Answer from the drawing. Dimensions are ordinates in mm from the lowest x, y and z of the part. A direction names the side the tool comes from. Give positions to 0.01 mm unless a question says otherwise; leave off trailing zeros. Write each loop counter-clockwise with the first axis right and the second up, starting at its lowest first coordinate (ties: lowest second). Pieces come first, ordered by that corner, then holes. Notation, with made-up numbers: (-18, 64.5) -> (-10, 64.5) arc R25 cw to (-10, 89.5) -> close; hole circle Ø4 at (73.25, 89.5). An arc over 180 degrees is marked (long way). Put each result on its own line as item: value. Start each with the question number.
1) A cutting plane is placed at C-C (y = 32). Write down the section's boundary in (x, z), then the cut area to 3 significant figures.
2) For a pull along Z with two mould halves and no side action, classify the marked faces 1, 2 and 3 as released by +Z, released by -Z, zero draft, split by the parting line, or undercut.
3) A cutting plane is placed at B-B (x = 54). Write down the section's boundary in (y, z), then the cut area to 3 significant figures.
4) A cutting plane is placed at D-D (z = 6). Give the number of separate pieces and of enclosed holes in the cut face, then the cut area to 3 significant figures.
5) A cutting plane is placed at A-A (y = 24.5). Write down the section's boundary in (x, z), then the cut area to 3 significant figures.
6) Find the intervals of material crossed by line 1 along Z through (x, y) = (54, 3); line 2 along X through (y, z) = (20, 8); line 3 along Y through (x, z) = (39.55, 15), in increasing order. Write a range as from..to.
7) For the marked faces 4, 5, 6 and 7, determine the directions among +Z, -Z, +X, -X, +Y, -Y from which every point of the face is accessible in a straight line to the end or side of a thin tool.
8) Flat-ended cylindrical pins translate along their axes: pin 1 Ø13 at (y, z) = (36, 15) entering from +X; pin 2 Ø6 at (y, z) = (13.5, 11.5) entering from -X; pin 3 Ø6.5 at (x, z) = (50.5, 19) entering from +Y. Find the tip coordinate at first contact, or state that the pin passes through.
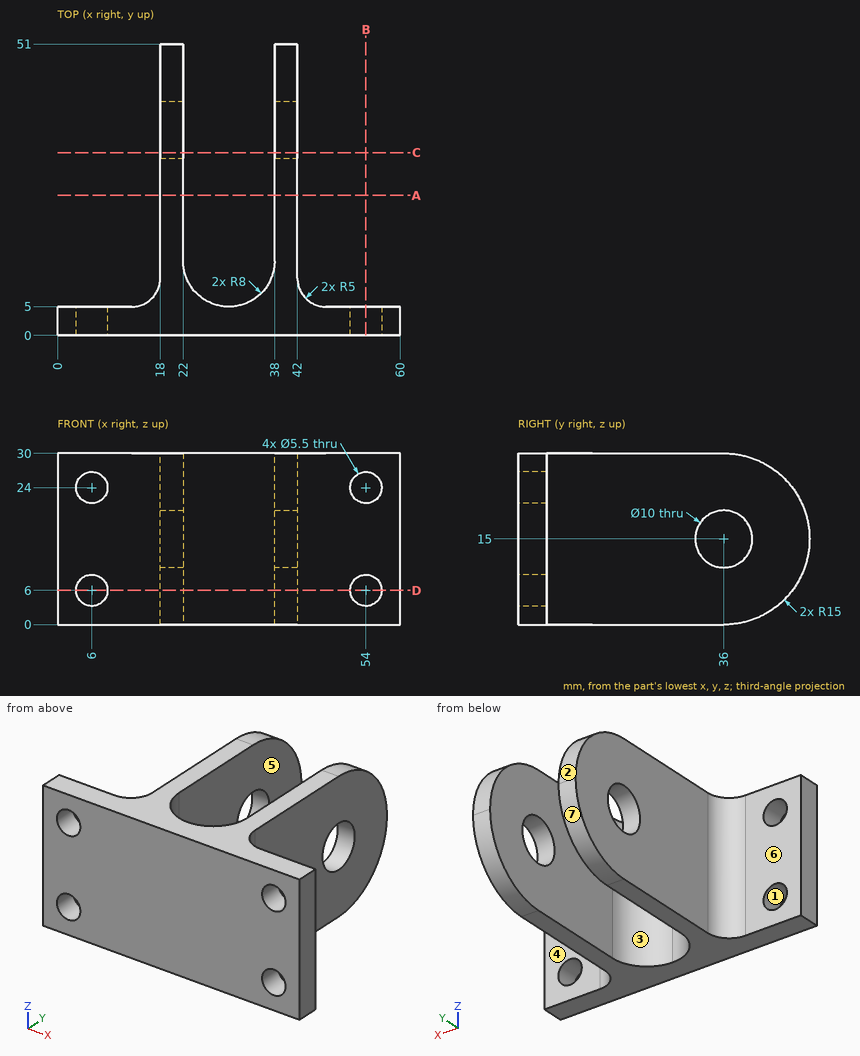
Reply:
1. outline: (18, 0) -> (22, 0) -> (22, 12) -> (18, 12) -> close; (18, 18) -> (22, 18) -> (22, 30) -> (18, 30) -> close; (38, 0) -> (42, 0) -> (42, 12) -> (38, 12) -> close; (38, 18) -> (42, 18) -> (42, 30) -> (38, 30) -> close
1. area: 192 mm2
2. face 1: undercut
2. face 2: released by +Z
2. face 3: zero draft
3. outline: (0, 0) -> (5, 0) -> (5, 3.25) -> (0, 3.25) -> close; (0, 8.75) -> (5, 8.75) -> (5, 21.25) -> (0, 21.25) -> close; (0, 26.75) -> (5, 26.75) -> (5, 30) -> (0, 30) -> close
3. area: 95.0 mm2
4. separate pieces: 3
4. enclosed holes: 0
4. area: 627 mm2
5. outline: (18, 0) -> (22, 0) -> (22, 30) -> (18, 30) -> close; (38, 0) -> (42, 0) -> (42, 30) -> (38, 30) -> close
5. area: 240 mm2
6. line 1: z = 0..3.25, 8.75..21.25, 26.75..30
6. line 2: x = 18..22, 38..42
6. line 3: y = 0..31, 41..51
7. face 4: +Z, -Z, +X, +Y
7. face 5: +Z, -Z, +Y
7. face 6: +Z, -Z, -X, +Y
7. face 7: -Z, +X, -X, +Y
8. pin 1: stops at x = 42
8. pin 2: stops at x = 18
8. pin 3: stops at y = 5
